```python
from build123d import *

# Parameters (mm, degrees)
EXTRUDE_1_DEPTH = 2.5


with BuildPart() as part:
    # 스케치1 → 보스-돌출1 (new, symmetric)
    with BuildSketch(Plane(origin=(0, 0, 0), x_dir=(1, 0, 0), z_dir=(0, 1, 0))):
        with BuildLine():
            Line((-49.642374512, -9.5), (-82.5, -9.5))
            Line((-82.5, -9.5), (-82.5, 9.5))
            Line((-82.5, 9.5), (-49.642374512, 9.5))
            ThreePointArc((-49.642374512, 9.5), (-39.177078252, 7.253737634), (-28.5, 6.5))
            Line((-28.5, 6.5), (28.5, 6.5))
            ThreePointArc((28.5, 6.5), (39.177078252, 7.253737634), (49.642374512, 9.5))
            Line((49.642374512, 9.5), (82.5, 9.5))
            Line((82.5, 9.5), (82.5, -9.5))
            Line((82.5, -9.5), (49.642374512, -9.5))
            ThreePointArc((49.642374512, -9.5), (39.177078252, -7.253737634), (28.5, -6.5))
            Line((28.5, -6.5), (-28.5, -6.5))
            ThreePointArc((-28.5, -6.5), (-39.177078252, -7.253737634), (-49.642374512, -9.5))
        make_face()
    extrude(amount=EXTRUDE_1_DEPTH, both=True)


solid = part.part
```
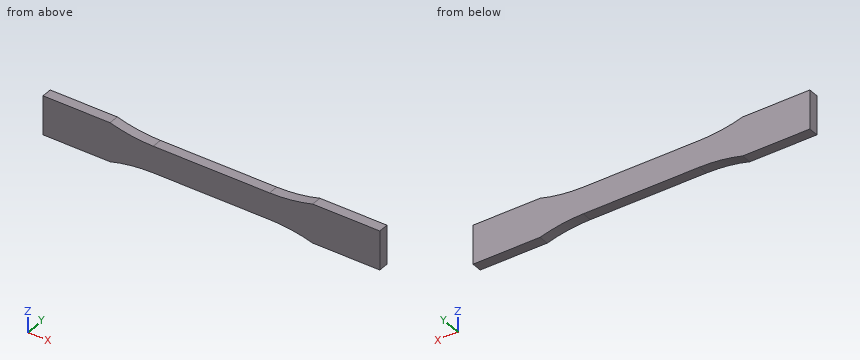
Here's how the part is built. I have some questions about the finished solid (model axes, mm). Round coordinates to 2 decimals unless told otherwise and drop trailing zeros. Write each loop counter-clockwise with the first axis right and the second up, starting at its lowest first coordinate (ties: lowest second). Pieces come first, ordered by that corner, then holes. Notation, with made-up numbers: M 5.25,63 L 60.25,63 A19 ccw 60.25,85 Z; hole C 36,-17.5 d5. An arc over 180 degrees is marked long. Answer as CSV lines item,"result". Start each with the question number.
1. Suppose I cut it at A-A on y = -0.45. Write out the boundary of the cut face in (x, z), then the cut area to 3 significant figures.
2. Suppose I cut it at C-C on x = 44. Write out the boundary of the cut face in (y, z), then the cut area to 3 significant figures.
3. Suppose I cut it at B-B on x = -21.5. Write out the boundary of the cut face in (y, z), then the cut area to 3 significant figures.
4. I need wall thicknesses on probe 1 along Z at (x, y) = (5, 1.05); probe 2 along Z at (x, y) = (48, -0.1). Which ranges of each line are inside material? Lowest first, please.
5. I'm going to push flat-ended pins straight in: pin 1 Ø2.5 at (x, y) = (-9.5, 0.5) entering from -Z; pin 2 Ø2.5 at (x, y) = (-12, -1) entering from +Z. Where does each tip first touch, or does it pass through?
Check result:
1,outline,"M -82.5,-9.5 L -49.64,-9.5 A76 cw -28.5,-6.5 L 28.5,-6.5 A76 cw 49.64,-9.5 L 82.5,-9.5 L 82.5,9.5 L 49.64,9.5 A76 cw 28.5,6.5 L -28.5,6.5 A76 cw -49.64,9.5 L -82.5,9.5 Z"
1,area,"2,620 mm2"
2,outline,"M -2.5,-8.1 L 2.5,-8.1 L 2.5,8.1 L -2.5,8.1 Z"
2,area,"81.0 mm2"
3,outline,"M -2.5,-6.5 L 2.5,-6.5 L 2.5,6.5 L -2.5,6.5 Z"
3,area,"65.0 mm2"
4,probe 1,"z = -6.5 to 6.5"
4,probe 2,"z = -9.04 to 9.04"
5,pin 1,"stops at z = -6.5"
5,pin 2,"stops at z = 6.5"
